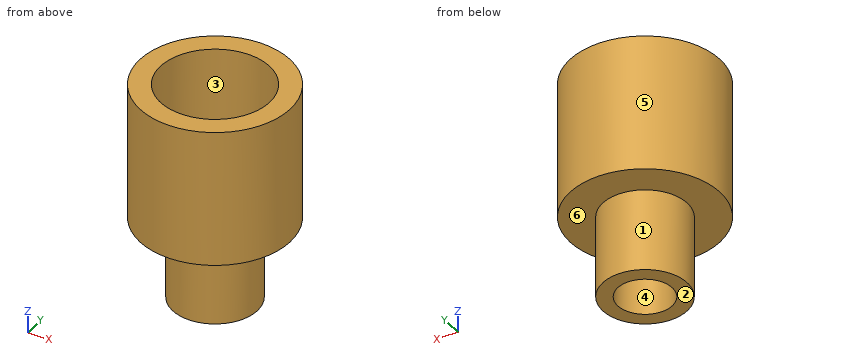
from build123d import *

# Parameters (mm, degrees)
F0_R     = 2.75
F0_R_2   = 2
F1_DEPTH = 5
F0_R_3   = 1.55
F2_DEPTH = 1
F0_R_4   = 1
F3_DEPTH = 3
F4_DEPTH = 1


with BuildPart() as f1:
    # F0 (on Top) → F1 (new body)
    with BuildSketch(Plane.XY):
        Circle(F0_R)
        Circle(F0_R_2, mode=Mode.SUBTRACT)
    extrude(amount=F1_DEPTH)

    # F0 (on Top) → F2 (join)
    with BuildSketch(Plane.XY):
        Circle(F0_R)
        Circle(F0_R_2, mode=Mode.SUBTRACT)
        Circle(F0_R_2)
        Circle(F0_R_3, mode=Mode.SUBTRACT)
    extrude(amount=F2_DEPTH)

    # F0 (on Top) → F3 (join)
    with BuildSketch(Plane.XY):
        Circle(F0_R_3)
        Circle(F0_R_4, mode=Mode.SUBTRACT)
    extrude(amount=-F3_DEPTH)

    # F0 (on Top) → F4 (join)
    with BuildSketch(Plane.XY):
        Circle(F0_R_3)
        Circle(F0_R_4, mode=Mode.SUBTRACT)
    extrude(amount=F4_DEPTH)


solid = f1.part
Source: CAD feature listing. Evaluate the final solid. Frame: model axes, mm. Face numbers are marked on the shaded views. A direction names the side the tool comes from. Round coordinates to 2 decimals unless told otherwise and drop trailing zeros. Loops run counter-clockwise (first coordinate to the right, second up) from the corner with the lowest first, then second, coordinate; pieces in that order, holes last.
Q1. Access query for the marked faces 5 and 6. Directions: +Z, -Z, +X, -X, +Y, -Y. A direction counts if a zero-diameter tool reaches every point of the face in a straight line with its end or side. Return the directions, or none.
Q2. Ray query, line 1 (Y direction, x = 0, z = -1.2); line 2 (Y direction, x = 0, z = 2.8); line 3 (Z direction, x = 1.3, y = -2.2). Return the intervals inside material, ascending.
Q3. Section C-C, the plane z = 4.25. Return loops of the section in (x, y), plus the area to 3 significant figures.
Q4. Section A-A, the plane y = 0. Return loops of the section in (x, z).
Q5. First-contact query: P1, Ø2, axis at y = -2, z = 2, coming from the -X side; P2, Ø1.2, axis at x = 0, y = 0, coming from the -Z side; P3, Ø3, axis at x = 0, y = 0, coming from the +Z side. Flat tips, straight axial feed; report the tip coordinate or a pass-through.
Q6. Section D-D, the plane x = -1.9. Return loops of the section in (y, z), plus the area to 3 significant figures.
Q7. Mould query, pull axis X, two halves, no side actions, for the marked faces 1, 2, 3 and 4. Classes: pulls with the +X half, pulls with the -X half, needs draft (parallel to the pull), parting line crosses it, or undercut.
Solutions:
1. face 5: +Z, -Z
1. face 6: -Z
2. line 1: y = -1.55 to -1, 1 to 1.55
2. line 2: y = -2.75 to -2, 2 to 2.75
2. line 3: z = 0 to 5
3. outline: circle Ø5.5 at (0, 0); hole circle Ø4 at (0, 0)
3. area: 11.2 mm2
4. outline: (-2.75, 0) - (-1.55, 0) - (-1.55, -3) - (-1, -3) - (-1, 1) - (-2, 1) - (-2, 5) - (-2.75, 5) - close; (1, -3) - (1.55, -3) - (1.55, 0) - (2.75, 0) - (2.75, 5) - (2, 5) - (2, 1) - (1, 1) - close
5. P1: stops at x = -2.56
5. P2: passes through
5. P3: stops at z = 1
6. outline: (-1.99, 0) - (1.99, 0) - (1.99, 5) - (0.62, 5) - (0.62, 1) - (-0.62, 1) - (-0.62, 5) - (-1.99, 5) - close
6. area: 14.9 mm2
7. face 1: parting line crosses it
7. face 2: needs draft
7. face 3: undercut
7. face 4: undercut
